Source: three-view drawing plus pictorial views. Frame: mm from the lowest corner of the part. Give positions to 0.01 mm unless a question says otherwise; leave off trailing zeros. Order: outer loops, then holes, each group sorted by start corner. A loop starts at its lowest first (then second) coordinate and runs counter-clockwise, first axis right, second up. Notation, with made-up numbers: (-8, 11) - (22, 11) arc R15 cw to (22, 29) - close; hole circle Ø2 at (-4.5, -0.5). An arc over 180 degrees is marked (long way). Use CSV: the item, a comma, the result in double quotes.
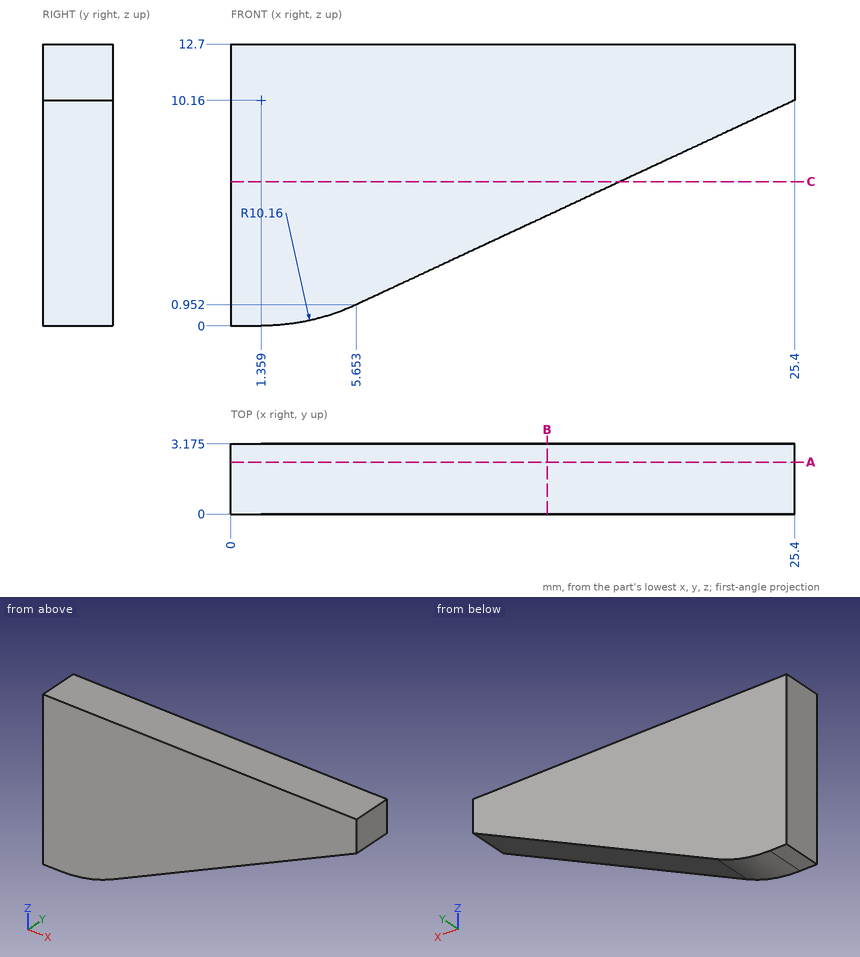
Item 1: Material intervals for line 1 (X direction, y = 2.9, z = 7.75) (1 decimal); line 2 (X direction, y = 1.9, z = 2); line 3 (Z direction, x = 23.25, y = 0.35), sorted ascending. Write a range as from..to.
Filled in:
line 1,"x = 0..20.2"
line 2,"x = 0..7.9"
line 3,"z = 9.16..12.7"
Item 2: First-contact query: pin 1 (2 mm diameter, centred on x = 8, z = 6.5, fed in from -Y). Flat tip, straight axial feed; report the tip coordinate or a pass-through.
Filled in:
pin 1,"stops at y = 0"
Item 3: Section B-B on x = 14.25. Return the cut outline in (y, z) (1 decimal), then the cut area to 3 significant figures.
Filled in:
outline,"(0, 5) - (3.2, 5) - (3.2, 12.7) - (0, 12.7) - close"
area,"24.6 mm2"
Item 4: Section A-A on y = 2.35. Return the cut outline in (x, z).
Filled in:
outline,"(0, 0) - (1.36, 0) arc R10.16 ccw to (5.65, 0.95) - (25.4, 10.16) - (25.4, 12.7) - (0, 12.7) - close"
Item 5: Section C-C on z = 6.5. Return the cut outline in (x, y) (1 decimal).
Filled in:
outline,"(0, 0) - (17.6, 0) - (17.6, 3.2) - (0, 3.2) - close"
